Can you work these out from the model? Positions are in its coordinate system, mm. Face numbers are marked on the shaded views. A direction names the side the tool comes from. Give positions to 0.01 mm unless a question says otherwise; leave off trailing zeros. Loops run counter-clockwise (first coordinate to the right, second up) from the corner with the lowest first, then second, coordinate; pieces in that order, holes last. Notation, with made-up numbers: (83.25, 37) -> (129.25, 37) arc R28 ccw to (129.25, 73) -> close; hole circle Ø8 at (-1.75, 57). An arc over 180 degrees is marked (long way). Return JSON: item names as keys, results as strings. Group by question number.
Q1. Suppose I cut it at C-C, the plane y = -1. Please give me the cut outline in (x, z), and give its area (3 significant figures).
Q2. Which directions (+Z, -Z, +X, -X, +Y, -Y) give clear straight access to the entire face, cutting with the end or side of a thin tool? Please do the marked faces 1, 2, 3 and 4.
Q3. Will these pins go through, and if not, where does the flat tip stop? pin 1 (1.5 mm diameter, centred on x = 20.5, y = -8, fed in from +Z); pin 2 (4 mm diameter, centred on x = -17, y = -11, fed in from -Z); pin 3 (6 mm diameter, centred on y = -12, z = 4.5, fed in from +X); pin 4 (3 mm diameter, centred on x = -31.5, y = -11, fed in from +Z).
Q4. I need wall thicknesses on line 1 along Y through (x, z) = (0, 7.25); line 2 along X through (y, z) = (10, 10); line 3 along X through (y, z) = (9, 12.25). Which ranges of each line are inside material? Lowest first, please. Write a range as [from, to].
Q5. Suppose I cut it at B-B, the plane x = 0. Please give me the cut outline in (y, z).
Q6. Suppose I cut it at A-A, the plane z = 6.35. Please give me the cut outline in (x, y), and give its area (3 significant figures).
Q7. Suppose I cut it at D-D, the plane x = -11.5. Please give me the cut outline in (y, z), and give its area (3 significant figures).
Q8. Thinking about a two-plate mould opening in Y: for the marked faces 5, 6 and 7, which applies, pulls with the +Y half, pulls with the -Y half, needs draft (parallel to the pull), parting line crosses it, or undercut?
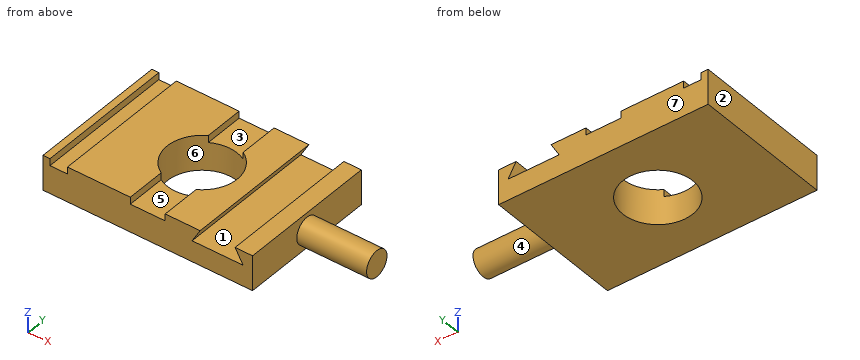
```python
from build123d import *

# Parameters (mm, degrees)
F0_W     = 76.2
F0_H     = 50.8
F0_R     = 12.7
F1_DEPTH = 12.7
F2_W     = 6.35
F2_H     = 50.8
F3_DEPTH = 2.54
F5_DEPTH = 50.801
F6_R     = 4.7625
F7_DEPTH = 25.4


with BuildPart() as f1:
    # F0 (on Top) → F1 (new body)
    with BuildSketch(Plane.XY):
        Rectangle(F0_W, F0_H)
        Circle(F0_R, mode=Mode.SUBTRACT)
    extrude(amount=F1_DEPTH)

    # F2 (on face) → F3 (cut)
    with BuildSketch(Plane.XY.offset(12.7)):
        with Locations((-32.385, 0)):
            Rectangle(F2_W, F2_H)
        with BuildLine():
            Line((6.35, 25.4), (-6.35, 25.4))
            Line((-6.35, 25.4), (-6.35, 10.9985226281))
            ThreePointArc((-6.35, 10.9985226281), (0, 12.7), (6.35, 10.9985226281))
            Line((6.35, 10.9985226281), (6.35, 25.4))
        make_face()
        with BuildLine():
            ThreePointArc((6.35, 10.9985226281), (0, 12.7), (-6.35, 10.9985226281))
            Line((-6.35, 10.9985226281), (-6.35, -10.9985226281))
            ThreePointArc((-6.35, -10.9985226281), (0, -12.7), (6.35, -10.9985226281))
            Line((6.35, -10.9985226281), (6.35, 10.9985226281))
        make_face()
        with BuildLine():
            Line((-6.35, -10.9985226281), (-6.35, -25.4))
            Line((-6.35, -25.4), (6.35, -25.4))
            Line((6.35, -25.4), (6.35, -10.9985226281))
            ThreePointArc((6.35, -10.9985226281), (0, -12.7), (-6.35, -10.9985226281))
        make_face()
    extrude(amount=-F3_DEPTH, mode=Mode.SUBTRACT)

    # F4 (on face) → F5 (cut, through all)
    with BuildSketch(Plane.XZ.offset(25.4)):
        Polygon((31.75, 12.7), (19.05, 12.7), (16.1170606325, 7.62), (34.6829393675, 7.62), align=None)
    extrude(amount=-F5_DEPTH, mode=Mode.SUBTRACT)

    # F6 (on face) → F7 (join)
    with BuildSketch(Plane.YZ.offset(38.1)):
        with Locations((0, 6.35)):
            Circle(F6_R)
    extrude(amount=F7_DEPTH)


solid = f1.part
```
Ans:
{
 "1": {"outline": "(-38.1, 0) -> (-12.66, 0) -> (-12.66, 12.7) -> (-29.21, 12.7) -> (-29.21, 10.16) -> (-35.56, 10.16) -> (-35.56, 12.7) -> (-38.1, 12.7) -> close; (12.66, 0) -> (38.1, 0) -> (38.1, 1.69) -> (63.5, 1.69) -> (63.5, 11.01) -> (38.1, 11.01) -> (38.1, 12.7) -> (31.75, 12.7) -> (34.68, 7.62) -> (16.12, 7.62) -> (19.05, 12.7) -> (12.66, 12.7) -> close", "area": "787 mm^2"},
 "2": {"face 1": "+Y, -Y", "face 2": "+Z, -Z, -X, +Y, -Y", "face 3": "+Z, +Y, -Y", "face 4": "+X"},
 "3": {"pin 1": "stops at z = 7.62", "pin 2": "stops at z = 0", "pin 3": "stops at x = 38.1", "pin 4": "stops at z = 10.16"},
 "4": {"line 1": "y = [-25.4, -12.7], [12.7, 25.4]", "line 2": "x = [-38.1, -7.83], [7.83, 17.49], [33.31, 38.1]", "line 3": "x = [-38.1, -35.56], [-29.21, -8.96], [8.96, 18.79], [32.01, 38.1]"},
 "5": {"outline": "(-25.4, 0) -> (-12.7, 0) -> (-12.7, 10.16) -> (-25.4, 10.16) -> close; (12.7, 0) -> (25.4, 0) -> (25.4, 10.16) -> (12.7, 10.16) -> close"},
 "6": {"outline": "(-38.1, -25.4) -> (38.1, -25.4) -> (38.1, -4.76) -> (63.5, -4.76) -> (63.5, 4.76) -> (38.1, 4.76) -> (38.1, 25.4) -> (-38.1, 25.4) -> close; hole circle Ø25.4 at (0, 0)", "area": "3,610 mm^2"},
 "7": {"outline": "(-25.4, 0) -> (-5.39, 0) -> (-5.39, 12.7) -> (-25.4, 12.7) -> close; (5.39, 0) -> (25.4, 0) -> (25.4, 12.7) -> (5.39, 12.7) -> close", "area": "508 mm^2"},
 "8": {"face 5": "needs draft", "face 6": "undercut", "face 7": "pulls with the +Y half"}
}
